Geometry: final body of the model. Coordinates: model frame, mm. A direction names the side the tool comes from. Give positions to 0.01 mm unless a question says otherwise; leave off trailing zeros. Loops run counter-clockwise (first coordinate to the right, second up) from the corner with the lowest first, then second, coordinate; pieces in that order, holes last.
Autodesk Inventor part; units mm, degrees
ref_plane "YZ Plane" through (0, 0, 0) normal (1, 0, 0) x (0, 1, 0)
ref_plane "XZ Plane" through (0, 0, 0) normal (0, 1, 0) x (-1, 0, 0)
ref_plane "XY Plane" through (0, 0, 0) normal (0, 0, 1) x (1, 0, 0)
sketch "Boceto1" plane through (0, 0, 0) normal (0, 1, 0) x (-1, 0, 0)
  line L0 (0.1, 0.1) -> (-0.1, 0.1)
  line L1 (-0.1, 0.1) -> (-0.1, -0.1)
  line L2 (-0.1, -0.1) -> (0.1, -0.1)
  line L3 (0.1, -0.1) -> (0.1, 0.1)
  point P0 (0, 0)
  dimension "L" = 0.2
  dimension "d1" = 0.2
  dimension "d2" = 0.1
  dimension "d3" = 0.1
extrude "Extrusión1" add sketch "Boceto1" along normal blind 11
sketch "Boceto2" plane through (0, 11, 0) normal (0, 1, 0) x (1, 0, 0)
  line L0 (-1.183, 1.017) -> (1.317, 1.017)
  line L1 (1.317, 1.017) -> (1.317, -1.183)
  line L2 (1.317, -1.183) -> (-1.183, -1.183)
  line L3 (-1.183, -1.183) -> (-1.183, 1.017)
  point P0 (0, 0)
  dimension "d6" = 2.2
  dimension "d7" = 2.5
extrude "Extrusión2" add sketch "Boceto2" against normal blind 1.6
ref_plane "Plano de trabajo1" through (0.067, 11, 1.183) normal (1, 0, 0) x (0, 0, -1)
ref_plane "Plano de trabajo2" through (-1.183, 11, 0.083) normal (0, 0, 1) x (1, 0, 0)
ref_plane "Plano de trabajo3" through (-1.183, 11, 0.083) normal (0, 0, 1) x (1, 0, 0)
ref_plane "Plano de trabajo4" through (0, 11, 0) normal (0, 1, 0) x (1, 0, 0)
sketch "Boceto3" plane through (0, 11, 0) normal (0, 1, 0) x (1, 0, 0)
  circle A0 centre (0.067, -0.083) radius 0.45
  line L0 (1.317, -1.183) -> (1.317, 1.017)
  line L1 (1.317, 1.017) -> (-1.183, 1.017)
  line L2 (-1.183, 1.017) -> (-1.183, -1.183)
  line L3 (-1.183, -1.183) -> (1.317, -1.183)
  point P0 (0, 0)
  dimension "d11" = 0.9
  dimension "d12" = 1.1
  dimension "d13" = 1.25
extrude "Extrusión3" add sketch "Boceto3" along normal blind 1.6 contours A0
sketch "Boceto4" plane through (0, 0, 0) normal (0, -1, 0) x (1, 0, 0)
  line L0 (0.1, 0.1) -> (0.1, -0.1)
  line L1 (-0.1, 0.1) -> (0.1, 0.1)
  line L2 (-0.1, -0.1) -> (-0.1, 0.1)
  line L3 (0.1, -0.1) -> (-0.1, -0.1)
  line L4 (0.1, -0.1) -> (0.1, 0.1)
  line L5 (0.1, 0.1) -> (-0.1, 0.1)
  line L6 (-0.1, 0.1) -> (-0.1, -0.1)
  line L7 (-0.1, -0.1) -> (0.1, -0.1)
  line L8 (0.1, -0.1) -> (0.1, 0.1)
  point P0 (0, 0)
extrude "Extrusión4" cut sketch "Boceto4" against normal blind 5
equation "\"d1\" = L"
properties part number "pata"
Item 1: Ray query, probe 1 along Y at (x, z) = (0.7, 0.5); probe 2 along X at (y, z) = (12.25, 0.05); probe 3 along Y at (x, z) = (0.2, 0). Return the intervals inside material, ascending.
Values follow:
probe 1: y = 9.4 to 11
probe 2: x = -0.38 to 0.52
probe 3: y = 9.4 to 12.6
Item 2: Pin query (flat end, axial travel): pin 1 (1.1 mm diameter, centred on x = 0.5, z = 0, fed in from -Y); pin 2 (1 mm diameter, centred on x = -0.5, z = -0.5, fed in from -Y). Return the tip coordinate at first contact, or that it passes through.
Values follow:
pin 1: stops at y = 5
pin 2: stops at y = 9.4
Item 3: Section query B-B on z = 0.75. Return loops of the section in (x, y).
Values follow:
outline: (-1.18, 9.4) - (1.32, 9.4) - (1.32, 11) - (-1.18, 11) - close
Item 4: Set-up query: faces 1 (the face through (0, 10, -1.017)), 2 (the face through (0.01, 11.79, 0.53)). Return all of +Z, -Z, +X, -X, +Y, -Y with unobstructed straight access to the full face (end or side cutting, diameter ignored); none if empty.
Values follow:
face 1: -Z, +X, -X, +Y, -Y
face 2: +Y
Item 5: Section query C-C on y = 8.75. Return loops of the section in (x, z), plus the area to 3 significant figures.
Values follow:
outline: (-0.1, -0.1) - (0.1, -0.1) - (0.1, 0.1) - (-0.1, 0.1) - close
area: 0.0400 mm2
Item 6: Section query D-D on z = 0.4. Return loops of the section in (x, y).
Values follow:
outline: (-1.18, 9.4) - (1.32, 9.4) - (1.32, 11) - (0.39, 11) - (0.39, 12.6) - (-0.25, 12.6) - (-0.25, 11) - (-1.18, 11) - close
Item 7: Section query A-A on x = 0.2. Return loops of the section in (y, z).
Values follow:
outline: (9.4, -1.02) - (11, -1.02) - (11, -0.35) - (12.6, -0.35) - (12.6, 0.51) - (11, 0.51) - (11, 1.18) - (9.4, 1.18) - close
